Read the model definition and answer for the solid it produces. Units are mm, in the model's axes. Face numbers are marked on the shaded views. A direction names the side the tool comes from. Round coordinates to 2 decimals unless told otherwise and drop trailing zeros. Order: outer loops, then holes, each group sorted by start corner. A loop starts at its lowest first (then second) coordinate and runs counter-clockwise, first axis right, second up. Notation, with made-up numbers: (1, 19) - (48, 19) arc R9 cw to (48, 35) - close; hole circle Ø3 at (37.25, -34). An arc over 180 degrees is marked (long way). Answer as a JSON object with one key per item and string values. Group by question number.
Q1. Given pin 1 Ø4 at (x, z) = (-12, 6.5) entering from -Y, flat-ended and moving along its own axis, determine where the tip first touches the part or whether it passes through.
Q2. A tool of negligible diameter and unlimited length cuts with its end or side. For the marked faces 1 and 2, from which of +Z, -Z, +X, -X, +Y, -Y can it reach the whole face along a straight path? Write none if from no direction.
Q3. A cutting plane is placed at C-C on x = -20.5. Determine the outline of the cut face in (y, z).
Q4. Consider line 1 (Y direction, x = -14.5, z = 3.25); line 2 (X direction, y = 31.5, z = 11.25). Determine where each line is inside the solid, lowest interval first.
Q5. A cutting plane is placed at A-A on z = 11.25. Determine the outline of the cut face in (x, y), and give its area (3 significant figures).
Q6. A cutting plane is placed at B-B on y = 63. Determine the outline of the cut face in (x, z), and give its area (3 significant figures).
Autodesk Inventor part; units mm, degrees
ref_plane "Work Plane1" through (-26.6941, 57.0071, 12.5) normal (0, 0, 1) x (1, 0, 0)
ref_plane "YZ Plane" through (0, 0, 0) normal (1, 0, 0) x (0, 1, 0)
ref_plane "XZ Plane" through (0, 0, 0) normal (0, 1, 0) x (-1, 0, 0)
sketch "Sketch2" plane through (0, 0, 0) normal (0, 0, 1) x (1, 0, 0)
  line L0 (0.6059, 79.2071) -> (0.6059, 64.0071)
  line L1 (-21.8941, 64.0071) -> (-21.8941, 79.2071)
  line L2 (-35.7896, 30.0586) -> (-39.3896, 30.0586)
  line L3 (-39.3896, 25.2586) -> (-35.7896, 25.2586)
  line L4 (-35.7896, 25.2586) -> (-39.3896, 25.2586)
  line L5 (-39.3896, 25.2586) -> (-39.3896, 68.8314)
  line L6 (-35.7896, 64.0071) -> (-35.7896, 25.2586)
  line L7 (0.6059, 64.0071) -> (-35.7896, 64.0071)
  line L8 (-39.3896, 64.0071) -> (-39.3896, 68.8314)
  line L9 (-39.3896, 68.8314) -> (0.6059, 68.8314)
  line L10 (0.6059, 68.8314) -> (0.6059, 64.0071)
  point P0 (0, 0)
ref_plane "Work Plane1" through (-26.6941, 57.0071, 12.5) normal (0, 0, 1) x (1, 0, 0)
extrude "Extrusion1" add sketch "Sketch2" along normal up to surface (12.5 mm away)
properties part number "frame2"
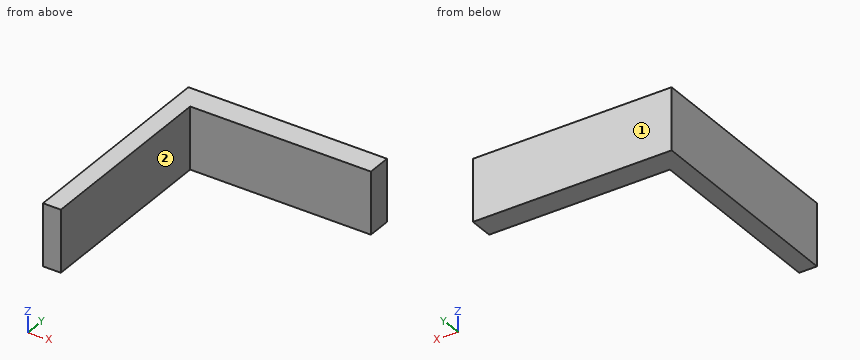
Result set:
{
 "1": {"pin 1": "stops at y = 64.01"},
 "2": {"face 1": "+Z, -Z, +X, -X, +Y", "face 2": "+Z, -Z, +X, -Y"},
 "3": {"outline": "(64.01, 0) - (68.83, 0) - (68.83, 12.5) - (64.01, 12.5) - close"},
 "4": {"line 1": "y = 64.01 to 68.83", "line 2": "x = -39.39 to -35.79"},
 "5": {"outline": "(-39.39, 25.26) - (-35.79, 25.26) - (-35.79, 64.01) - (0.61, 64.01) - (0.61, 68.83) - (-39.39, 68.83) - close", "area": "332 mm²"},
 "6": {"outline": "(-39.39, 0) - (-35.79, 0) - (-35.79, 12.5) - (-39.39, 12.5) - close", "area": "45.0 mm²"}
}
